Read the model definition and answer for the solid it produces. Units are mm, in the model's axes. Face numbers are marked on the shaded views. A direction names the side the tool comes from. Round coordinates to 2 decimals unless told otherwise and drop trailing zeros. Write each loop counter-clockwise with the first axis right and the second up, starting at its lowest first coordinate (ties: lowest second). Pieces come first, ordered by that corner, then holes.
Autodesk Inventor part; units mm, degrees
ref_plane "YZ Plane" through (0, 0, 0) normal (1, 0, 0) x (0, 1, 0)
ref_plane "XZ Plane" through (0, 0, 0) normal (0, 1, 0) x (-1, 0, 0)
ref_plane "XY Plane" through (0, 0, 0) normal (0, 0, 1) x (1, 0, 0)
sketch "スケッチ1" plane through (0, 0, 0) normal (0, 0, 1) x (1, 0, 0)
  line L0 (-235, 10.2629) -> (65, 10.2629)
  line L1 (65, 10.2629) -> (65, 5.2629)
  line L2 (65, 5.2629) -> (-235, 5.2629)
  line L3 (-235, 5.2629) -> (-235, 10.2629)
  line L4 (-235, 10.2629) -> (65, 5.2629) construction
  line L5 (65, 10.2629) -> (-235, 5.2629) construction
  point P0 (0, 0)
  point P1 (-85, 7.7629)
  dimension "d0" = 300
  dimension "d1" = 5
extrude "押し出し1" add sketch "スケッチ1" along normal blind 600
sketch "スケッチ2" plane through (-235, 5.2629, 0) normal (0, -1, 0) x (1, 0, 0)
  line L0 (50, 0) -> (250, 0)
  line L1 (250, 0) -> (250, 600)
  line L2 (250, 600) -> (50, 600)
  line L3 (50, 600) -> (50, 0)
  line L4 (300, 0) -> (0, 0)
  line L5 (0, 0) -> (0, 600)
  point P0 (235, 0)
  dimension "d4" = 200
  dimension "d5" = 600
  dimension "d6" = 0
  dimension "d7" = 50
extrude "押し出し2" add sketch "スケッチ2" along normal blind 55
sketch "スケッチ3" plane through (-235, -49.7371, 0) normal (0, -1, 0) x (1, 0, 0)
  line L0 (-60, -20) -> (360, -20)
  line L1 (360, -20) -> (360, 620)
  line L2 (360, 620) -> (-60, 620)
  line L3 (-60, 620) -> (-60, -20)
  line L4 (0, 0) -> (300, 0)
  line L5 (0, 0) -> (0, 600)
  point P0 (235, 0)
  dimension "d10" = 420
  dimension "d11" = 640
  dimension "d12" = 20
  dimension "d13" = 60
extrude "押し出し3" add sketch "スケッチ3" along normal blind 10
sketch "スケッチ4" plane through (-235, -49.7371, 0) normal (0, 1, 0) x (1, 0, 0)
  line L0 (-55, 2.2049) -> (355, 2.2049)
  line L1 (355, 2.2049) -> (355, 0)
  line L2 (355, 0) -> (-55, 0)
  line L3 (-55, 0) -> (-55, 2.2049)
  line L4 (-60, -620) -> (-60, 20)
  line L5 (-60, 20) -> (360, 20)
  line L6 (-55, -603) -> (355, -603)
  line L7 (355, -603) -> (355, -600)
  line L8 (355, -600) -> (-55, -600)
  line L9 (-55, -600) -> (-55, -603)
  line L10 (360, -620) -> (-60, -620)
  point P0 (235, 0)
  dimension "d16" = 410
  dimension "d17" = 5
  dimension "d18" = 20
  dimension "d19" = 410
  dimension "d20" = 3
  dimension "d21" = 20
  dimension "d22" = 5
extrude "押し出し4" cut sketch "スケッチ4" against normal blind 5
sketch "スケッチ5" plane through (15, 5.2629, 600) normal (1, 0, 0) x (0, 0, -1)
  line L0 (600, 0) -> (600, -55)
  line L1 (0, 0) -> (600, 0)
  line L2 (600, 0) -> (600, -55)
  line L3 (600, -55) -> (0, -55)
  line L4 (0, -55) -> (0, 0)
  point P0 (600, -5.2629)
extrude "押し出し5" cut sketch "スケッチ5" against normal blind 2
sketch "スケッチ6" plane through (-185, 5.2629, 0) normal (-1, 0, 0) x (0, 0, 1)
  line L0 (0, 0) -> (600, 0)
  line L1 (-20, -55) -> (620, -55)
  line L2 (0, 0) -> (600, 0)
  line L3 (600, 0) -> (600, -55)
  line L4 (600, -55) -> (0, -55)
  line L5 (0, -55) -> (0, 0)
  point P0 (0, -5.2629)
extrude "押し出し6" cut sketch "スケッチ6" against normal blind 2
sketch "スケッチ7" plane through (-235, -59.7371, 0) normal (0, -1, 0) x (1, 0, 0)
  circle A0 centre (150, 300) radius 100
  line L0 (-60, 620) -> (-60, -20)
  line L1 (-60, -20) -> (360, -20)
  point P0 (235, 0)
  dimension "d29" = 200
  dimension "d30" = 210
  dimension "d31" = 320
extrude "押し出し7" add sketch "スケッチ7" along normal blind 100
sketch "スケッチ8" plane through (-85, -159.7371, 300) normal (0, -1, 0) x (1, 0, 0)
  circle A0 centre (0, 0) radius 52.5
  point P0 (85, -300)
  dimension "d34" = 105
extrude "押し出し8" add sketch "スケッチ8" along normal blind 50
sketch "スケッチ9" plane through (-85, -209.7371, 300) normal (0, -1, 0) x (1, 0, 0)
  arc A0 (52.5, 0) -> (-52.5, 0) centre (0, 0) ccw
  line L0 (52.5, 0) -> (-52.5, 0)
  point P0 (85, -300)
  dimension "d37" = 105
extrude "押し出し9" add sketch "スケッチ9" along normal blind 50
properties part number "nasel_stand"
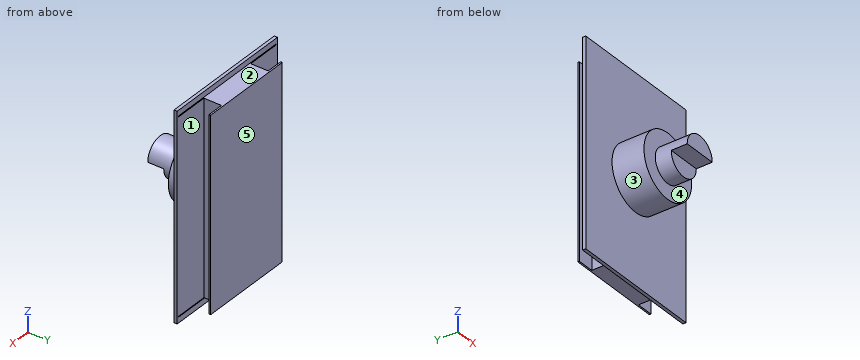
Q1. Which of the six approach directions +Z, -Z, +X, -X, +Y, -Y give full straight-line access (tool end or side, diameter ignored) to the marked faces 4 and 5?
Verdict:
face 4: -Y
face 5: +Z, -Z, +X, -X, +Y
Q2. Section C-C (y = -13) is taken. Determine the outline of the cut face in (x, z), then the cut area to 3 significant figures.
Verdict:
outline: (-183, 0) - (13, 0) - (13, 600) - (-183, 600) - close
area: 118,000 mm2
Q3. Section B-B (z = 171.5) is taken. Determine the outline of the cut face in (x, y).
Verdict:
outline: (-295, -59.74) - (125, -59.74) - (125, -49.74) - (13, -49.74) - (13, 5.26) - (65, 5.26) - (65, 10.26) - (-235, 10.26) - (-235, 5.26) - (-183, 5.26) - (-183, -49.74) - (-295, -49.74) - close
Q4. Section A-A (x = -194) is taken. Determine the outline of the cut face in (y, z), then the cut area to 3 significant figures.
Verdict:
outline: (-59.74, -20) - (-49.74, -20) - (-49.74, -2.2) - (-54.74, -2.2) - (-54.74, 0) - (-49.74, 0) - (-49.74, 600) - (-54.74, 600) - (-54.74, 603) - (-49.74, 603) - (-49.74, 620) - (-59.74, 620) - close; (5.26, 0) - (10.26, 0) - (10.26, 600) - (5.26, 600) - close
area: 9,370 mm2
Q5. Flat-ended cylindrical pins translate along their axes: pin 1 Ø1.5 at (x, y) = (-34.5, -142.5) entering from +Z; pin 2 Ø15.5 at (x, z) = (-214, 284) entering from -Y; pin 3 Ø2.5 at (y, z) = (7.5, 233.5) entering from -X. Find the tip coordinate at first contact, or state that the pin passes through.
Verdict:
pin 1: stops at z = 386.75
pin 2: stops at y = -59.74
pin 3: stops at x = -235
Q6. Determine the mould class of the marked faces 1, 2 and 3 for opening direction X: pulls with the +X half, pulls with the -X half, needs draft (parallel to the pull), parting line crosses it, or undercut.
Verdict:
face 1: needs draft
face 2: undercut
face 3: parting line crosses it
Q7. Section D-D (x = -85) is taken. Determine the outline of the cut face in (y, z).
Verdict:
outline: (-259.74, 300) - (-209.74, 300) - (-209.74, 247.5) - (-159.74, 247.5) - (-159.74, 200) - (-59.74, 200) - (-59.74, -20) - (-49.74, -20) - (-49.74, -2.2) - (-54.74, -2.2) - (-54.74, 0) - (10.26, 0) - (10.26, 600) - (-54.74, 600) - (-54.74, 603) - (-49.74, 603) - (-49.74, 620) - (-59.74, 620) - (-59.74, 400) - (-159.74, 400) - (-159.74, 352.5) - (-259.74, 352.5) - close
Q8. Straight lines are drawn through the part: probe 1 along Y at (x, z) = (-205, 295); probe 2 along Y at (x, z) = (81.5, 41.5); probe 3 along X at (y, z) = (-43, 496.5). For each, find the intervals that lie inside material, in ascending order.
Verdict:
probe 1: y = -59.74 to -49.74, 5.26 to 10.26
probe 2: y = -59.74 to -49.74
probe 3: x = -183 to 13
